from build123d import *

# Parameters (mm, degrees)
F0_R     = 4
F0_R_2   = 3.5
F0_R_3   = 1.5
F0_R_4   = 2
F0_R_5   = 2.5
F1_DEPTH = 0.5
F2_SIZE  = 4


with BuildPart() as f1:
    # F0 (on Top) → F1 (new body, symmetric)
    with BuildSketch(Plane.XY):
        Polygon((-92.5, 128.2), (-92.5, 0), (-92.5, -128.2), (-60, -128.2), (-60, -142.5), (0, -142.5), (60, -142.5), (60, -128.2), (92.5, -128.2), (92.5, 0), (92.5, 128.2), (60, 128.2), (60, 142.5), (0, 142.5), (-60, 142.5), (-60, 128.2), align=None)
        with Locations((-84.5, -120)):
            Circle(F0_R, mode=Mode.SUBTRACT)
        with Locations((-63.25, -92.5)):
            Circle(F0_R_2, mode=Mode.SUBTRACT)
        with Locations((-63, -62.2)):
            Circle(F0_R_3, mode=Mode.SUBTRACT)
        with Locations((48, -130)):
            Circle(F0_R_4, mode=Mode.SUBTRACT)
        with Locations((84.5, -120)):
            Circle(F0_R, mode=Mode.SUBTRACT)
        with Locations((63.25, -92.5)):
            Circle(F0_R_2, mode=Mode.SUBTRACT)
        with Locations((63, -62.2)):
            Circle(F0_R_3, mode=Mode.SUBTRACT)
        with Locations((-63, 62.2)):
            Circle(F0_R_3, mode=Mode.SUBTRACT)
        with Locations((-42.5, 27.5)):
            Circle(F0_R_5, mode=Mode.SUBTRACT)
        with Locations((-84.5, 120)):
            Circle(F0_R, mode=Mode.SUBTRACT)
        with Locations((17.5, 27.5)):
            Circle(F0_R_5, mode=Mode.SUBTRACT)
        with Locations((63, 62.2)):
            Circle(F0_R_3, mode=Mode.SUBTRACT)
        with Locations((84.5, 120)):
            Circle(F0_R, mode=Mode.SUBTRACT)
    extrude(amount=F1_DEPTH, both=True)

    # F2
    f2_edges = [f1.edges().sort_by_distance(p)[0] for p in [
        (-92.5, 128.2, 0),
        (-60, 142.5, 0),
        (60, 142.5, 0),
        (92.5, 128.2, 0),
        (92.5, -128.2, 0),
        (60, -142.5, 0),
        (-60, -142.5, 0),
        (-92.5, -128.2, 0),
    ]]
    chamfer(f2_edges, length=F2_SIZE)


solid = f1.part
CAD build for the part. Positions are in the model's coordinates, mm. Give positions to 0.01 mm unless a question says otherwise; leave off trailing zeros. Write each loop counter-clockwise with the first axis right and the second up, starting at its lowest first coordinate (ties: lowest second). Pieces come first, ordered by that corner, then holes. Notation, with made-up numbers: M 50,81.5 L 75,81.5 A21 cw 75,92.5 Z; hole C 69.25,-34 d4. An arc over 180 degrees is marked long. Put each result on its own line as item: value. Start each with the question number.
(1) Flat gauge pins, fed straight in: pin 1 Ø0.5 at (x, z) = (75.5, 0) entering from +Y; pin 2 Ø0.5 at (y, z) = (135.5, 0) entering from +X. Where does each tip first touch, or does it go through?
(2) Band-saw the part on A-A, the plane y = 120. Write the cut outline in (x, z), and give its area (3 significant figures).
(3) Probe L1, parallel to Y at x = 84.5, z = -0.15; L2, parallel to Y at x = 63.25, z = 0; L3, parallel to Y at x = 81, z = 0.25. List the from-to ranges inside material, lowest first.
(4) Band-saw the part on B-B, the plane z = -0.1. Give the number of separate pieces and of enclosed holes in the cut face, and give its area (3 significant figures).
(5) Mould opens along X. For faces 1 (the face through (60.473, -94.63, -0.007)), 2 (the face through (-1, 2, 0.5)) say: +X half, -X half, draft (parallel to the pull), parting line (faces both ways), or undercut.
Response values:
1. pin 1: stops at y = 128.2
1. pin 2: stops at x = 60
2. outline: M -92.5,-0.5 L -88.5,-0.5 L -88.5,0.5 L -92.5,0.5 Z; M -80.5,-0.5 L 80.5,-0.5 L 80.5,0.5 L -80.5,0.5 Z; M 88.5,-0.5 L 92.5,-0.5 L 92.5,0.5 L 88.5,0.5 Z
2. area: 169 mm2
3. L1: y = -128.2 to -124, -116 to 116, 124 to 128.2
3. L2: y = -128.2 to -96, -89 to -63.68, -60.72 to 60.72, 63.68 to 128.2
3. L3: y = -128.2 to -121.94, -118.06 to 118.06, 121.94 to 128.2
4. separate pieces: 1
4. enclosed holes: 13
4. area: 50,400 mm2
5. face 1: undercut
5. face 2: draft
